Can you work these out from the model? Positions are in its coordinate system, mm. Face numbers are marked on the shaded views. A direction names the side the tool comes from. Coordinates: 2 decimals unless noted, no trailing zeros. Order: outer loops, then holes, each group sorted by start corner. A loop starts at its lowest first (then second) coordinate and runs counter-clockwise, first axis right, second up. Notation, with made-up numbers: (64.25, -35) -> (69.25, -35) arc R17 cw to (69.25, -2) -> close; hole circle Ø8 at (15, 24.25). An arc over 180 degrees is marked (long way). Return JSON: item names as keys, results as strings. Group by question number.
1) Thinking about a two-plate mould opening in Y: for the marked faces 1, 2 and 3, which applies, +Y half, -Y half, draft (parallel to the pull), parting line (faces both ways), or undercut?
2) If we section it at B-B, the plane x = -3.5: Please give me the cut outline in (y, z).
3) If we section it at A-A, the plane z = 3.65: Please give me the cut outline in (x, y).
4) If we section it at D-D, the plane y = 3.55: Please give me the cut outline in (x, z), then the cut area to 3 significant figures.
5) If I drill on probe 1 along X at (y, z) = (3.95, 3.2); probe 2 along X at (y, z) = (1.5, 1.85); probe 3 along Y at (x, z) = (-4.5, 1), over which ranges is the centre line in solid material (lowest first)? Write a range as from..to.
6) For the marked faces 4 and 5, which set-ups out of +Z, -Z, +X, -X, +Y, -Y let a thin tool reach every point of the face, with its end or its side?
7) If we section it at C-C, the plane y = 1: Please give me the cut outline in (x, z).
8) For pin 1 (1.5 mm diameter, centred on y = 2, z = 3, fed in from -X), with a flat end and sliding along its axis, tell me the tip position at first contact or that it passes through.
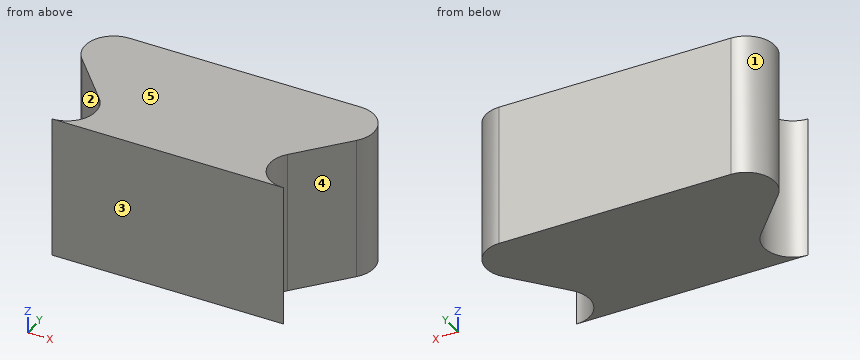
from build123d import *

# Parameters (mm, degrees)
F1_DEPTH = 5


with BuildPart() as f1:
    # F0 (on Top) → F1 (new body)
    with BuildSketch(Plane.XY):
        with BuildLine():
            Line((0, 5), (-4, 5))
            ThreePointArc((-4, 5), (-4.912871, 4.408248), (-4.745356, 3.333333))
            Line((-4.745356, 3.333333), (-3.254644, 1.666667))
            ThreePointArc((-3.254644, 1.666667), (-3.087129, 0.591752), (-4, 0))
            Line((-4, 0), (0, 0))
            Line((0, 0), (0, 5))
        make_face()
    extrude(amount=F1_DEPTH)

    # F2: F1 across face


with BuildPart() as f1_1:
    add(f1.part)
    add(f1.part.mirror(Plane(origin=(0, 2.5, 2.5), x_dir=(0, 1, 0), z_dir=(1, 0, 0))))


solid = f1_1.part
Result sheet:
{
 "1": {"face 1": "parting line", "face 2": "undercut", "face 3": "-Y half"},
 "2": {"outline": "(0, 0) -> (0.13, 0) -> (0.13, 5) -> (0, 5) -> close; (1.94, 0) -> (5, 0) -> (5, 5) -> (1.94, 5) -> close"},
 "3": {"outline": "(-4.75, 3.33) -> (-3.25, 1.67) arc R1 cw to (-4, 0) -> (4, 0) arc R1 cw to (3.25, 1.67) -> (4.75, 3.33) arc R1 ccw to (4, 5) -> (-4, 5) arc R1 ccw to start"},
 "4": {"outline": "(-4.89, 0) -> (4.89, 0) -> (4.89, 5) -> (-4.89, 5) -> close", "area": "48.9 mm2"},
 "5": {"probe 1": "x = -5..5", "probe 2": "x = -3.13..3.13", "probe 3": "y = 3.06..4.87"},
 "6": {"face 4": "+Z, -Z, +X", "face 5": "+Z, +X, -X, +Y, -Y"},
 "7": {"outline": "(-3, 0) -> (3, 0) -> (3, 5) -> (-3, 5) -> close"},
 "8": {"pin 1": "stops at x = -4.22"}
}
